Autodesk Inventor part; units mm, degrees
ref_plane "YZ Plane" through (0, 0, 0) normal (1, 0, 0) x (0, 1, 0)
ref_plane "XZ Plane" through (0, 0, 0) normal (0, 1, 0) x (-1, 0, 0)
ref_plane "XY Plane" through (0, 0, 0) normal (0, 0, 1) x (1, 0, 0)
sketch "Sketch1" plane through (0, 0, 0) normal (0, 0, 1) x (1, 0, 0)
  line L0 (-15.5217, 12.1376) -> (24.4783, 12.1376)
  line L1 (24.4783, 12.1376) -> (24.4783, -11.8624)
  line L2 (24.4783, -11.8624) -> (-15.5217, -11.8624)
  line L3 (-15.5217, -11.8624) -> (-15.5217, 12.1376)
  point P0 (0, 0)
  dimension "d0" = 40
  dimension "d1" = 24
extrude "Extrusion1" add sketch "Sketch1" along normal blind 29
sketch "Sketch2" plane through (-15.5217, -11.8624, 0) normal (-1, 0, 0) x (0, 0, 1)
  line L0 (0, 0) -> (0, 24)
  line L1 (0, 0) -> (29, 0)
  line L2 (0, 24) -> (1.5, 24)
  line L3 (1.5, 24) -> (1.5, 0)
  line L4 (1.5, 0) -> (0, 0)
  line L5 (0, 0) -> (0, 24)
  line L6 (0, 24) -> (29, 24)
  line L7 (29, 24) -> (27.5, 24)
  line L8 (27.5, 24) -> (27.5, 0)
  line L9 (27.5, 0) -> (29, 0)
  line L10 (29, 0) -> (29, 24)
  line L11 (1.5, 24) -> (27.5, 24)
  line L12 (27.5, 24) -> (27.5, 0)
  line L13 (27.5, 0) -> (1.5, 0)
  line L14 (1.5, 0) -> (1.5, 24)
  point P0 (0, 11.8624)
  dimension "d4" = 1.5
  dimension "d5" = 1.5
  dimension "d6" = 24
extrude "Extrusion2" cut sketch "Sketch2" against normal blind 38.5 contours L3 L6 L8 L1
sketch "Sketch3" plane through (24.4783, -11.8624, 0) normal (1, 0, 0) x (0, 0, -1)
  line L0 (0, 24) -> (-29, 24)
  line L1 (0, 24) -> (0, 0)
  line L2 (-29, 0) -> (-29, 24)
  circle A0 centre (-14.5, 12) radius 1.5
  circle A1 centre (-14.5, 12) radius 2.5
  line L3 (0, 24) -> (-12.574, 13.5939)
  line L4 (-16.426, 10.4061) -> (-29, 0)
  line L5 (-29, 24) -> (-16.426, 13.5939)
  line L6 (-12.574, 10.4061) -> (0, 0)
  point P0 (0, 11.8624)
  dimension "d9" = 3
  dimension "d10" = 5
extrude "Extrusion3" add sketch "Sketch3" along normal blind 0.5 contours A1
sketch "Sketch4" plane through (24.4783, -11.8624, 0) normal (1, 0, 0) x (0, 0, -1)
  line L0 (0, 24) -> (0, 0)
  line L1 (0, 0) -> (-29, 0)
  line L2 (0, 24) -> (-29, 0)
  line L3 (0, 24) -> (-29, 24)
  line L4 (-29, 24) -> (0, 0)
  circle A0 centre (-14.5, 12) radius 1.5
  circle A1 centre (-14.5, 12) radius 1.5
  point P0 (0, 11.8624)
  dimension "d13" = 3
extrude "Extrusion4" cut sketch "Sketch4" against normal blind 1.5 contours A0 L4 L2 | L2 L4 A0 | A0 L2 L4 | L2 A0 L4
sketch "Sketch5" plane through (-15.5217, -11.8624, 1.5) normal (0, 0, 1) x (1, 0, 0)
  line L0 (0, 24) -> (40, 24)
  line L1 (0, 24) -> (1, 24)
  line L2 (1, 24) -> (1, 0)
  line L3 (1, 0) -> (0, 0)
  line L4 (0, 0) -> (0, 24)
  line L5 (1, 24) -> (5.5, 24)
  line L6 (5.5, 24) -> (5.5, 0)
  line L7 (5.5, 0) -> (1, 0)
  line L8 (1, 0) -> (1, 24)
  point P0 (15.5217, 11.8624)
  dimension "d16" = 1
  dimension "d17" = 24
  dimension "d18" = 4.5
  dimension "d19" = 24
extrude "Extrusion5" add sketch "Sketch5" along normal blind 26 contours L0 L6 L7 L2
sketch "Sketch6" plane through (-14.5217, -11.8624, 1.5) normal (-1, 0, 0) x (0, 0, 1)
  line L0 (26, 24) -> (26, 0)
  line L1 (-1.5, 24) -> (27.5, 24)
  line L2 (26, 0) -> (0, 0)
  circle A0 centre (13, 12) radius 6
  line L3 (0, 24) -> (8.5912, 16.0697)
  line L4 (17.4088, 7.9303) -> (26, 0)
  line L5 (26, 24) -> (17.4088, 16.0697)
  line L6 (8.5912, 7.9303) -> (0, 0)
  point P0 (-1.5, 11.8624)
  dimension "d22" = 12
extrude "Extrusion6" cut sketch "Sketch6" against normal blind 4.5 contours A0
sketch "Sketch7" plane through (22.9783, -11.8624, 0) normal (-1, 0, 0) x (0, 0, 1)
  line L0 (27.5, 0) -> (1.5, 0)
  line L1 (27.5, 24) -> (1.5, 0)
  line L2 (1.5, 0) -> (1.5, 24)
  line L3 (1.5, 24) -> (27.5, 0)
  circle A0 centre (14.5, 12) radius 2.5
  circle A1 centre (14.5, 12) radius 12
  point P0 (0, 11.8624)
extrude "Extrusion7" add sketch "Sketch7" along normal blind 1 contours A1 L1 A0 L3 | L3 A0 L1 A1 | A1 L3 A0 L1 | A1 L1 A0 L3
fillet "Fillet1" radius 1.5 1 edges at (24.4783, 0.1376, 29)
fillet "Fillet2" radius 1.5 1 edges at (24.4783, 0.1376, 0)
sketch "Sketch8" plane through (0, 0, 29) normal (0, 0, 1) x (1, 0, 0)
  line L0 (-15.5217, -11.8624) -> (-15.5217, 12.1376)
  line L1 (-15.5217, 12.1376) -> (-5.5217, 12.1376)
  line L2 (-5.5217, 12.1376) -> (-5.5217, -11.8624)
  line L3 (-5.5217, -11.8624) -> (-15.5217, -11.8624)
  line L4 (-15.5217, -11.8624) -> (-15.5217, 12.1376)
  line L5 (-15.5217, 12.1376) -> (-5.5217, 12.1376)
  line L6 (-7.0217, -9.3624) -> (-15.5217, -9.3624)
  line L7 (-15.5217, -9.3624) -> (-15.5217, 12.1376)
  line L8 (-5.5217, -11.8624) -> (-15.5217, -11.8624)
  line L9 (-15.5217, -11.8624) -> (-15.5217, 9.6376)
  line L10 (-15.5217, 9.6376) -> (-7.0217, 9.6376)
  line L11 (-5.5217, 9.6376) -> (-5.5217, -11.8624)
  circle A0 centre (-5.5217, 9.6376) radius 1.5
  circle A1 centre (-5.5217, -9.3624) radius 1.5
  line L12 (-5.5217, 12.1376) -> (-5.5217, 9.6376)
  line L13 (-5.5217, 8.1376) -> (-5.5217, -9.3624)
  point P0 (0, 0)
  dimension "d35" = 3
  dimension "d29" = 10
  dimension "d30" = 24
  dimension "d31" = 10
  dimension "d32" = 21.5
  dimension "d33" = 21.5
  dimension "d34" = 3
extrude "Extrusion8" cut sketch "Sketch8" against normal blind 29 contours A1 L2 | L2 A1 | A0 L2 | L2 A0
sketch "Sketch9" plane through (0, 0, 29) normal (0, 0, 1) x (1, 0, 0)
  line L0 (-15.5217, 12.1376) -> (-15.5217, -11.8624)
  line L1 (-15.5217, 12.1376) -> (10.9783, 12.1376)
  line L2 (10.9783, 12.1376) -> (10.9783, -9.3624)
  line L3 (10.9783, -9.3624) -> (-15.5217, -9.3624)
  line L4 (-15.5217, -9.3624) -> (-15.5217, 12.1376)
  line L5 (10.9783, 12.1376) -> (10.9783, 10.0118)
  circle A0 centre (10.9783, -9.3624) radius 1.5
  circle A1 centre (10.9783, 9.6376) radius 1.5
  point P0 (0, 0)
  dimension "d38" = 26.5
  dimension "d39" = 3
  dimension "d40" = 3
extrude "Extrusion9" cut sketch "Sketch9" against normal blind 29 contours A0 L2 L3 | L3 L2 A0 | A1 L2 | L2 A1
sketch "Sketch10" plane through (22.9783, 0.1376, 14.5) normal (-1, 0, 0) x (0, 0, 1)
  circle A0 centre (0, 0) radius 1.5
  circle A1 centre (0, 0) radius 2.5
  point P0 (-14.5, -0.1376)
  dimension "d43" = 5
extrude "Extrusion10" add sketch "Sketch10" along normal blind 1
Geometry: final body of the model. Coordinates: model frame, mm. A direction names the side the tool comes from. Round coordinates to 2 decimals unless told otherwise and drop trailing zeros. Order: outer loops, then holes, each group sorted by start corner. A loop starts at its lowest first (then second) coordinate and runs counter-clockwise, first axis right, second up. Notation, with made-up numbers: (-15, -15) -> (27, -15) arc R25 ccw to (27, 19) -> close; hole circle Ø4 at (-39, -21.5). An arc over 180 degrees is marked (long way). Use one line per item in the form item = value. Start each with the question number.
1. Draft query along X for faces 1 (the face through (-15, 0, 1.5)), 2 (the face through (22.978, 2, 27)), 3 (the face through (-15.522, 0, 28)). Return one class per face: pulls with the +X half, pulls with the -X half, needs draft (parallel to the pull), parting line crosses it, or undercut.
2. Cut plane D-D (y = 3.5). Return the cut outline in (x, z), then the cut area to 3 significant figures.
3. Reachability of faces 4 (the face through (-14.522, 6, 11)), 5 (the face through (6, 0, 27.5)), 6 (the face through (-12.303, -2.16, 20.042)), 7 (the face through (22.49, -0.39, 2.51)) from +Z, -Z, +X, -X, +Y, -Y: full face, straight path, thin tool, end or side. Return the list, or none.
4. Line query: probe 1 along Z at (x, y) = (4.5, -10.25); probe 2 along X at (y, z) = (7.25, 11.25); probe 3 along Y at (x, z) = (-11.25, 14.5). Output: solid intervals per line, ascending.
5. Cut plane A-A (x = 1.5). Return the cut outline in (y, z), then the cut area to 3 significant figures.
6. Cut plane B-B (z = 17.5). Return the cut outline in (x, y).
7. Cut plane C-C (z = 22.5). Return the cut outline in (x, y), then the cut area to 3 significant figures.
8. Pin query (flat end, axial travel): pin 1 Ø1.8 at (y, z) = (0.14, 14.5) entering from +X; pin 2 Ø12 at (y, z) = (2.5, 8.5) entering from +X; pin 3 Ø10.5 at (y, z) = (5, 19) entering from -X; pin 4 Ø4 at (y, z) = (0.14, 14.5) entering from -X. Return the tip coordinate at first contact, or that it passes through.
Solution:
q1.face_1 = needs draft
q1.face_2 = undercut
q1.face_3 = pulls with the -X half
q2.outline = (-15.52, 0) -> (22.98, 0) arc R1.5 ccw to (24.48, 1.5) -> (24.48, 27.5) arc R1.5 ccw to (22.98, 29) -> (-15.52, 29) -> (-15.52, 27.5) -> (-14.52, 27.5) -> (-14.52, 19.47) -> (-10.02, 19.47) -> (-10.02, 27.5) -> (22.98, 27.5) -> (22.98, 26.02) -> (21.98, 26.02) -> (21.98, 2.98) -> (22.98, 2.98) -> (22.98, 1.5) -> (-10.02, 1.5) -> (-10.02, 9.53) -> (-14.52, 9.53) -> (-14.52, 1.5) -> (-15.52, 1.5) -> close
q2.area = 253 mm^2
q3.face_4 = -X, +Y, -Y
q3.face_5 = +Y, -Y
q3.face_6 = -X
q3.face_7 = none
q4.probe_1 = 0 to 1.5, 27.5 to 29
q4.probe_2 = -14.52 to -10.02, 21.98 to 24.48
q4.probe_3 = -11.86 to -5.86, 6.14 to 12.14
q5.outline = (-11.86, 0) -> (12.14, 0) -> (12.14, 1.5) -> (-11.86, 1.5) -> close; (-11.86, 27.5) -> (12.14, 27.5) -> (12.14, 29) -> (-11.86, 29) -> close
q5.area = 72.0 mm^2
q6.outline = (-14.52, -11.86) -> (-10.02, -11.86) -> (-10.02, -5.06) -> (-14.52, -5.06) -> close; (-14.52, 5.33) -> (-10.02, 5.33) -> (-10.02, 12.14) -> (-14.52, 12.14) -> close; (21.98, -11.48) -> (22.98, -11.48) -> (22.98, -11.86) -> (24.48, -11.86) -> (24.48, 12.14) -> (22.98, 12.14) -> (22.98, 11.76) -> (21.98, 11.76) -> close
q7.outline = (-14.52, -11.86) -> (-10.02, -11.86) -> (-10.02, 12.14) -> (-14.52, 12.14) -> close; (21.98, -8.81) -> (22.98, -8.81) -> (22.98, -11.86) -> (24.48, -11.86) -> (24.48, 12.14) -> (22.98, 12.14) -> (22.98, 9.08) -> (21.98, 9.08) -> close
q7.area = 162 mm^2
q8.pin_1 = through
q8.pin_2 = 24.98
q8.pin_3 = -14.52
q8.pin_4 = 21.98
